from build123d import *

# Parameters (mm, degrees)
F1_DEPTH    = 15
F2_R        = 2
F3_T1_DEPTH = 31


# Not quite as in the source:
# - a fillet or chamfer that OpenCascade refuses, or shapes differently, is made with other operations: its cross-section is extruded or revolved along the edge and cut away or added


with BuildPart() as f1:
    # F0 (on Top) → F1 (new body)
    with BuildSketch(Plane.XY):
        Polygon((0, 40), (0, 0), (28.0349999666, 0), (28.0349999666, 10), (10, 10), (10, 40), align=None)
        with BuildLine():
            Line((28.0349999666, 10), (28.0349999666, 0))
            ThreePointArc((28.0349999666, 0), (33.0349999666, 5), (28.0349999666, 10))
        make_face()
    extrude(amount=F1_DEPTH)

    # F2
    f2_edges = [f1.edges().sort_by_distance(p)[0] for p in [
        (10, 25, 15),
        (19.0175, 10, 15),
        (14.0175, 0, 0),
        (10, 40, 7.5),
        (0, 40, 7.5),
        (0, 0, 7.5),
        (0, 20, 0),
        (0, 20, 15),
        (10, 25, 0),
        (14.0175, 0, 15),
        (33.035, 5, 0),
        (33.035, 5, 15),
        (19.0175, 10, 0),
    ]]
    fillet(f2_edges, radius=F2_R)

    # F3: fillet of radius 5 on 4 edges, made by hand

    # F3_s2 → F3_t1 (cut)
    with BuildSketch(Plane.YZ.offset(-10.5)):
        with BuildLine():
            ThreePointArc((40, 5), (38.5355339059, 1.4644660941), (35, 0))
            Line((35, 0), (40, 0))
            Line((40, 0), (40, 5))
        make_face()
        with BuildLine():
            ThreePointArc((40, 10), (38.5355339059, 13.5355339059), (35, 15))
            Line((35, 15), (40, 15))
            Line((40, 15), (40, 10))
        make_face()
    extrude(amount=F3_T1_DEPTH, mode=Mode.SUBTRACT)


solid = f1.part
Could you check a few things on this model? Use its own coordinates, in mm. A direction names the side the tool comes from. Give positions to 0.01 mm unless a question says otherwise; leave off trailing zeros. Order: outer loops, then holes, each group sorted by start corner. A loop starts at its lowest first (then second) coordinate and runs counter-clockwise, first axis right, second up.
1. Suppose I cut it at C-C (z = 7). Write out the boundary of the cut face in (x, y) (3 decimals), plus the area to 3 significant figures.
Answers below:
outline: (0, 2) arc R2 ccw to (2, 0) - (28.035, 0) arc R5 ccw to (28.035, 10) - (10, 10) - (10, 38) arc R2 ccw to (8, 40) - (2, 40) arc R2 ccw to (0, 38) - close
area: 617 mm2
2. I need wall thicknesses on L1, parallel to X at y = 14, z = 4.25; L2, parallel to Z at x = 8.5, y = 21. Which ranges of each line are inside material? Lowest first, please.
Answers below:
L1: x = 0 to 10
L2: z = 0.06 to 14.94
3. Suppose I cut it at B-B (x = 3). Write out the boundary of the cut face in (y, z).
Answers below:
outline: (0, 2) arc R2 ccw to (2, 0) - (35, 0) arc R5 ccw to (40, 5) - (40, 10) arc R5 ccw to (35, 15) - (2, 15) arc R2 ccw to (0, 13) - close
4. For pin 1 (8 mm diameter, centred on y = 23, z = 7.5, fed in from +X); pin 2 (3.5 mm diameter, centred on x = 20, z = 5.5, fed in from +Y); pin 3 (3 mm diameter, centred on x = 11, y = 31.5, fed in from +Z), each with a flat end and sliding along its axis, tell me the tip position at first contact or that it passes through.
Answers below:
pin 1: stops at x = 10
pin 2: stops at y = 10
pin 3: stops at z = 14.32
5. Suppose I cut it at A-A (y = 19.5). Write out the boundary of the cut face in (x, z).
Answers below:
outline: (0, 2) arc R2 ccw to (2, 0) - (8, 0) arc R2 ccw to (10, 2) - (10, 13) arc R2 ccw to (8, 15) - (2, 15) arc R2 ccw to (0, 13) - close
6. Which directions (+Z, -Z, +X, -X, +Y, -Y) give clear straight access to the entire face, cutting with the end or side of a thin tool? Please do faces 1 (the flat face through (19, 10, 7)), 2 (the cylindrical face through (15.2, 0.57, 0.6)), 3 (the cylindrical face through (9.43, 23.48, 14.4)), 4 (the cylindrical face through (9.43, 23.48, 0.6)), 5 (the flat face through (7, 11, 0)).
Answers below:
face 1: +Z, -Z, +X, +Y
face 2: -Z, +X, -X, -Y
face 3: +Z, +X, +Y
face 4: -Z, +X, +Y
face 5: -Z, +X, -X, +Y, -Y
